Geometry: final body of the model. Coordinates: model frame, mm. Round coordinates to 2 decimals unless told otherwise and drop trailing zeros. Order: outer loops, then holes, each group sorted by start corner. A loop starts at its lowest first (then second) coordinate and runs counter-clockwise, first axis right, second up. Notation, with made-up numbers: M -8,80 L 39,80 A23 ccw 39,99 Z; hole C 9,70 d4. An arc over 180 degrees is marked long. Put each result on its own line as item: value. Start each with the question number.
1) Section A-A, the plane y = 0. Return loops of the section in (x, z), then the cut area to 3 significant figures.
2) Material intervals for probe 1 along Y at (x, z) = (0, -0.75); probe 2 along Y at (x, z) = (-4.75, -0.5); probe 3 along X at (y, z) = (-0.5, 0.55), sorted ascending. Write a range as [from, to].
3) Draft query along X for faces 1 (the cylindrical face through (7.2, -0.6, -0.5)), 2 (the cylindrical face through (11.923, 3.755, 0.014)), 3 (the flat face through (2.5, 2.8, -1.5)). Return one class per face: pulls with the +X half, pulls with the -X half, needs draft (parallel to the pull), parting line crosses it, or undercut.
4) Section C-C, the plane z = -0.25. Count the separate pieces of the cut face and the enclosed holes in it, then the cut area to 3 significant figures.
5) First-contact query: P1, Ø1.5, axis at x = 7, z = 0, coming from the +Y side; P2, Ø3, axis at x = -8, y = 0, coming from the +Z side; P3, Ø1, axis at x = -9.5, z = 0.5, coming from the -Y side. Flat tips, straight axial feed; report the tip coordinate or a pass-through.
from build123d import *

# Parameters (mm, degrees)
SKETCH_1_R      = 12.5
SKETCH_1_R_2    = 1
SKETCH_1_R_3    = 1.5
SKETCH_1_R_4    = 3.5
EXTRUDE_1_DEPTH = 1.5
CHAMFER_2_SIZE  = 1
CHAMFER_1_SIZE  = 0.5


with BuildPart() as part:
    # 草图1 → 凸台-拉伸1 (new, symmetric)
    with BuildSketch(Plane.XY):
        Circle(SKETCH_1_R)
        with Locations((0, 8)):
            Circle(SKETCH_1_R_2, mode=Mode.SUBTRACT)
        with Locations((8, 0)):
            Circle(SKETCH_1_R_2, mode=Mode.SUBTRACT)
        with Locations((0, -8)):
            Circle(SKETCH_1_R_2, mode=Mode.SUBTRACT)
        with Locations((-8, 0)):
            Circle(SKETCH_1_R_2, mode=Mode.SUBTRACT)
        with Locations((-4.242640687, 4.242640687)):
            Circle(SKETCH_1_R_3, mode=Mode.SUBTRACT)
        Circle(SKETCH_1_R_4, mode=Mode.SUBTRACT)
        with Locations((4.242640687, 4.242640687)):
            Circle(SKETCH_1_R_3, mode=Mode.SUBTRACT)
        with Locations((4.242640687, -4.242640687)):
            Circle(SKETCH_1_R_3, mode=Mode.SUBTRACT)
        with Locations((-4.242640687, -4.242640687)):
            Circle(SKETCH_1_R_3, mode=Mode.SUBTRACT)
    extrude(amount=EXTRUDE_1_DEPTH, both=True)

    # 倒角2
    chamfer_2_edges = [part.edges().sort_by_distance(p)[0] for p in [
        (-1, -8, 1.5),
        (-9, 0, 1.5),
        (-1, 8, 1.5),
        (7, 0, 1.5),
    ]]
    chamfer(chamfer_2_edges, length=CHAMFER_2_SIZE)

    # 倒角1
    chamfer_1_edges = [part.edges().sort_by_distance(p)[0] for p in [
        (-12.5, 0, -1.5),
        (-12.5, 0, 1.5),
    ]]
    chamfer(chamfer_1_edges, length=CHAMFER_1_SIZE)


solid = part.part
Result sheet:
1. outline: M -12.5,-1 L -12,-1.5 L -9,-1.5 L -9,0.5 L -10,1.5 L -12,1.5 L -12.5,1 Z; M -7,-1.5 L -3.5,-1.5 L -3.5,1.5 L -6,1.5 L -7,0.5 Z; M 3.5,-1.5 L 7,-1.5 L 7,0.5 L 6,1.5 L 3.5,1.5 Z; M 9,-1.5 L 12,-1.5 L 12.5,-1 L 12.5,1 L 12,1.5 L 10,1.5 L 9,0.5 Z
1. area: 39.5 mm2
2. probe 1: y = [-12.5, -9], [-7, -3.5], [3.5, 7], [9, 12.5]
2. probe 2: y = [-11.56, -5.65], [-2.83, 2.83], [5.65, 11.56]
2. probe 3: x = [-12.49, -8.92], [-7.08, -3.46], [3.46, 7.08], [8.92, 12.49]
3. face 1: undercut
3. face 2: parting line crosses it
3. face 3: needs draft
4. separate pieces: 1
4. enclosed holes: 9
4. area: 412 mm2
5. P1: stops at y = 10.83
5. P2: stops at z = 1
5. P3: stops at y = -8.67
